```python
from build123d import *

# Parameters (mm, degrees)
SKETCH1_R           = 2.15
BOSS_EXTRUDE1_DEPTH = 3
SKETCH2_R           = 2
CUT_EXTRUDE1_DEPTH  = 289.872749062
SKETCH3_R           = 3.175
CUT_EXTRUDE2_DEPTH  = 289.872749062
SKETCH4_W           = 127
SKETCH4_H           = 64.740069581
CUT_EXTRUDE3_DEPTH  = 289.872749062
SKETCH5_W           = 304.8
SKETCH5_H           = 67.289955289
CUT_EXTRUDE4_DEPTH  = 289.872749062
SKETCH6_R           = 2
CUT_EXTRUDE5_DEPTH  = 260.625171507
SKETCH7_R           = 3.175
CUT_EXTRUDE6_DEPTH  = 260.625171507
CUT_EXTRUDE7_DEPTH  = 260.625171507
FILLET1_R           = 2.54
FILLET2_R           = 2.54


with BuildPart() as part:
    # Sketch1 → Boss-Extrude1 (new body)
    with BuildSketch(Plane(origin=(0, 0, 0), x_dir=(1, 0, 0), z_dir=(0, 1, 0))):
        with BuildLine():
            Line((-126.953423408, -0.978024545), (172.766576592, -0.978024545))
            ThreePointArc((172.766576592, -0.978024545), (174.562627816, -1.721973321), (175.306576592, -3.518024545))
            Line((175.306576592, -3.518024545), (175.306576592, -227.038024545))
            ThreePointArc((175.306576592, -227.038024545), (174.562627816, -228.834075769), (172.766576592, -229.578024545))
            Line((172.766576592, -229.578024545), (-126.953423408, -229.578024545))
            ThreePointArc((-126.953423408, -229.578024545), (-128.749474632, -228.834075769), (-129.493423408, -227.038024545))
            Line((-129.493423408, -227.038024545), (-129.493423408, -3.518024545))
            ThreePointArc((-129.493423408, -3.518024545), (-128.749474632, -1.721973321), (-126.953423408, -0.978024545))
        make_face()
        with Locations(Location((3.856576592, -23.978144226, 0), (0, 0, 270))):
            Circle(SKETCH1_R, mode=Mode.SUBTRACT)
        with Locations(Location((41.956576592, -23.978144226, 0), (0, 0, 270))):
            Circle(SKETCH1_R, mode=Mode.SUBTRACT)
        with Locations(Location((3.856576592, -63.602144226, 0), (0, 0, 270))):
            Circle(SKETCH1_R, mode=Mode.SUBTRACT)
        with Locations(Location((41.956576592, -63.602144226, 0), (0, 0, 270))):
            Circle(SKETCH1_R, mode=Mode.SUBTRACT)
        with Locations(Location((3.856576592, -93.828144226, 0), (0, 0, 270))):
            Circle(SKETCH1_R, mode=Mode.SUBTRACT)
        with Locations(Location((41.956576592, -93.828144226, 0), (0, 0, 270))):
            Circle(SKETCH1_R, mode=Mode.SUBTRACT)
        with Locations(Location((3.856576592, -133.452144226, 0), (0, 0, 270))):
            Circle(SKETCH1_R, mode=Mode.SUBTRACT)
        with Locations(Location((41.956576592, -133.452144226, 0), (0, 0, 270))):
            Circle(SKETCH1_R, mode=Mode.SUBTRACT)
    extrude(amount=BOSS_EXTRUDE1_DEPTH)

    # Sketch2 → Cut-Extrude1 (cut, through all)
    with BuildSketch(Plane(origin=(0, 0, 0), x_dir=(-1, 0, 0), z_dir=(0, -1, 0))):
        with Locations(Location((21.543423408, -77.178024545, 0), (0, 0, 90))):
            Circle(SKETCH2_R)
        with Locations(Location((-67.356576592, -77.178024545, 0), (0, 0, 270))):
            Circle(SKETCH2_R)
        with Locations(Location((21.543423408, -127.978024545, 0), (0, 0, 270))):
            Circle(SKETCH2_R)
        with Locations(Location((-67.356576592, -127.978024545, 0), (0, 0, 90))):
            Circle(SKETCH2_R)
    extrude(amount=-CUT_EXTRUDE1_DEPTH, mode=Mode.SUBTRACT)

    # Sketch3 → Cut-Extrude2 (cut, through all)
    with BuildSketch(Plane(origin=(0, 0, 0), x_dir=(-1, 0, 0), z_dir=(0, -1, 0))):
        with Locations(Location((-48.306576592, -77.456208611, 0), (0, 0, 90))):
            Circle(SKETCH3_R)
        with Locations(Location((2.493423408, -77.456208611, 0), (0, 0, 90))):
            Circle(SKETCH3_R)
        with Locations(Location((2.493423408, -146.036208611, 0), (0, 0, 90))):
            Circle(SKETCH3_R)
        with Locations(Location((-48.306576592, -146.036208611, 0), (0, 0, 90))):
            Circle(SKETCH3_R)
    extrude(amount=-CUT_EXTRUDE2_DEPTH, mode=Mode.SUBTRACT)

    # Sketch4 → Cut-Extrude3 (cut, through all)
    with BuildSketch(Plane.XZ):
        with Locations((-71.073423408, 32.107989755)):
            Rectangle(SKETCH4_W, SKETCH4_H)
    extrude(amount=-CUT_EXTRUDE3_DEPTH, mode=Mode.SUBTRACT)

    # Sketch5 → Cut-Extrude4 (cut, through all)
    with BuildSketch(Plane.XZ):
        with Locations((22.906576592, 225.12300219)):
            Rectangle(SKETCH5_W, SKETCH5_H)
    extrude(amount=-CUT_EXTRUDE4_DEPTH, mode=Mode.SUBTRACT)

    # Sketch6 → Cut-Extrude5 (cut, through all)
    with BuildSketch(Plane(origin=(0, 0, 0), x_dir=(-1, 0, 0), z_dir=(0, -1, 0))):
        with Locations(Location((5.608304381, -133.452144226, 0), (0, 0, 90))):
            Circle(SKETCH6_R)
        with Locations(Location((-51.406576592, -94.452144226, 0), (0, 0, 90))):
            Circle(SKETCH6_R)
        with BuildLine():
            Line((-171.306576592, -2.978024545), (-169.806576592, -2.978024545))
            ThreePointArc((-169.806576592, -2.978024545), (-167.806576592, -4.978024545), (-169.806576592, -6.978024545))
            Line((-169.806576592, -6.978024545), (-171.306576592, -6.978024545))
            ThreePointArc((-171.306576592, -6.978024545), (-173.306576592, -4.978024545), (-171.306576592, -2.978024545))
        make_face()
        with BuildLine():
            Line((-132.356576592, -59.978024545), (-130.806576592, -59.978024545))
            ThreePointArc((-130.806576592, -59.978024545), (-128.806576592, -61.978024545), (-130.806576592, -63.978024545))
            Line((-130.806576592, -63.978024545), (-132.356576592, -63.978024545))
            ThreePointArc((-132.356576592, -63.978024545), (-134.356576592, -61.978024545), (-132.356576592, -59.978024545))
        make_face()
    extrude(amount=-CUT_EXTRUDE5_DEPTH, mode=Mode.SUBTRACT)

    # Sketch7 → Cut-Extrude6 (cut, through all)
    with BuildSketch(Plane.XZ):
        with Locations(Location((149.906576592, 77.178024545, 0), (0, 0, 270))):
            Circle(SKETCH7_R)
        with Locations(Location((-116.793423408, 89.878024545, 0), (0, 0, 270))):
            Circle(SKETCH7_R)
        with Locations(Location((-116.793423408, 178.778024545, 0), (0, 0, 270))):
            Circle(SKETCH7_R)
        with Locations(Location((162.606576592, 178.778024545, 0), (0, 0, 270))):
            Circle(SKETCH7_R)
    extrude(amount=-CUT_EXTRUDE6_DEPTH, mode=Mode.SUBTRACT)

    # Sketch8 → Cut-Extrude7 (cut, through all)
    with BuildSketch(Plane(origin=(0, 0, 0), x_dir=(-1, 0, 0), z_dir=(0, -1, 0))):
        with BuildLine():
            Line((-12.746576592, -83.806208611), (-33.066576592, -83.806208611))
            ThreePointArc((-33.066576592, -83.806208611), (-34.862627816, -83.062259835), (-35.606576592, -81.266208611))
            Line((-35.606576592, -81.266208611), (-35.606576592, -73.646208611))
            ThreePointArc((-35.606576592, -73.646208611), (-34.862627816, -71.850157387), (-33.066576592, -71.106208611))
            Line((-33.066576592, -71.106208611), (-12.746576592, -71.106208611))
            ThreePointArc((-12.746576592, -71.106208611), (-10.950525368, -71.850157387), (-10.206576592, -73.646208611))
            Line((-10.206576592, -73.646208611), (-10.206576592, -81.266208611))
            ThreePointArc((-10.206576592, -81.266208611), (-10.950525368, -83.062259835), (-12.746576592, -83.806208611))
        make_face()
    extrude(amount=-CUT_EXTRUDE7_DEPTH, mode=Mode.SUBTRACT)

    # Fillet1
    fillet1_edges = [part.edges().sort_by_distance(p)[0] for p in [
        (175.306576592, 1.5, 191.478024545),
        (-129.493423408, 1.5, 191.478024545),
    ]]
    fillet(fillet1_edges, radius=FILLET1_R)

    # Fillet2
    fillet2_edges = [part.edges().sort_by_distance(p)[0] for p in [
        (-7.573423408, 1.5, 64.478024545),
        (-129.493423408, 1.5, 64.478024545),
        (-7.573423408, 1.5, 0.978024545),
    ]]
    fillet(fillet2_edges, radius=FILLET2_R)


solid = part.part
```
Could you check a few things on this model? Use its own coordinates, in mm. Give positions to 0.01 mm unless a question says otherwise; leave off trailing zeros. Write each loop counter-clockwise with the first axis right and the second up, starting at its lowest first coordinate (ties: lowest second). Pieces come first, ordered by that corner, then holes. Notation, with made-up numbers: (83.25, 18) -> (100.25, 18) arc R19 cw to (100.25, 36) -> close; hole circle Ø3 at (84, 34). An arc over 180 degrees is marked (long way). Write each question's results on one line, items separated by ' | '.
1. Will this pin go through, and if not, where does the flat tip stop? pin 1 Ø0.9 at (x, y) = (-70, 2) entering from -Z.
Check sheet entries:
pin 1: stops at z = 64.48
2. I want a section at C-C, the plane z = 30. Write out the boundary of the cut face in (x, y).
Check sheet entries:
outline: (-7.57, 0) -> (175.31, 0) -> (175.31, 3) -> (-7.57, 3) -> close
3. I want a section at A-A, the plane x = 27. Write out the boundary of the cut face in (y, z), then the cut area to 3 significant figures.
Check sheet entries:
outline: (0, 0.98) -> (3, 0.98) -> (3, 71.11) -> (0, 71.11) -> close; (0, 83.81) -> (3, 83.81) -> (3, 191.48) -> (0, 191.48) -> close | area: 533 mm²
4. I want a section at D-D, the plane y = 2.1. Count the separate pieces of the cut face and the enclosed holes in it, then the cut area to 3 significant figures.
Check sheet entries:
separate pieces: 1 | enclosed holes: 25 | area: 49,500 mm²
5. I need wall thicknesses on L1, parallel to X at y = 0.3, z = 94; L2, parallel to Z at x = -117, y = 1.2; L3, parallel to X at y = 0.9, z = 181. Which ranges of each line are inside material? Lowest first, please.
Check sheet entries:
L1: x = -129.49 to 1.71, 6 to 39.81, 44.1 to 49.46, 53.35 to 175.31 | L2: z = 64.48 to 86.71, 93.05 to 175.61, 181.95 to 191.48 | L3: x = -129.49 to -119.06, -114.53 to 160.34, 164.87 to 175.31
6. If we mould it in two halves opening along Z, with no side actions, what happens to faces 1 (the cylindrical face through (-114.65, 1.48, 92.22)), 2 (the flat face through (25, 3, 95)), 3 (the cylindrical face through (148.691, 1.479, 74.245))? For each: released by +Z, released by -Z, zero draft, split by the parting line, or undercut.
Check sheet entries:
face 1: undercut | face 2: zero draft | face 3: undercut
7. I want a section at B-B, the plane x = -68.5. Write out the boundary of the cut face in (y, z), then the cut area to 3 significant figures.
Check sheet entries:
outline: (0, 64.48) -> (3, 64.48) -> (3, 191.48) -> (0, 191.48) -> close | area: 381 mm²
